For this review, take the finished solid that the model builds, in its own axes (mm). Face numbers are marked on the shaded views. A direction names the side the tool comes from. Round coordinates to 2 decimals unless told otherwise and drop trailing zeros. Order: outer loops, then holes, each group sorted by start corner. A loop starts at its lowest first (then second) coordinate and runs counter-clockwise, first axis right, second up. Notation, with made-up numbers: M 58.5,11 L 98.5,11 A30 ccw 98.5,48 Z; hole C 43,86 d9. An arc over 180 degrees is marked long. Answer in a Markdown table with one row per item. Add a question column.
```python
from build123d import *

# Parameters (mm, degrees)
SKETCH_1_R          = 18
EXTRUDE_1_DEPTH     = 1
SKETCH_2_R          = 8
EXTRUDE_2_DEPTH     = 17
SKETCH_3_R          = 2
EXTRUDE_3_DEPTH     = 3
SKETCH_4_R          = 5
CUT_EXTRUDE_1_DEPTH = 8
SKETCH_5_W          = 4.070351758
SKETCH_5_H          = 5.859394111
CUT_EXTRUDE_2_DEPTH = 0.5


with BuildPart() as part:
    # Эскиз1 → Бобышка-Вытянуть1 (new body)
    with BuildSketch(Plane(origin=(0, 0, 0), x_dir=(1, 0, 0), z_dir=(0, 1, 0))):
        with Locations(Location((0, 0, 0), (0, 0, 270))):
            Circle(SKETCH_1_R)
    extrude(amount=EXTRUDE_1_DEPTH)

    # Эскиз2 → Бобышка-Вытянуть2 (add)
    with BuildSketch(Plane(origin=(0, 1, 0), x_dir=(1, 0, 0), z_dir=(0, 1, 0))):
        with Locations(Location((0, 0, 0), (0, 0, 270))):
            Circle(SKETCH_2_R)
    extrude(amount=EXTRUDE_2_DEPTH)

    # Эскиз3 → Бобышка-Вытянуть3 (add)
    with BuildSketch(Plane(origin=(0, 18, 0), x_dir=(1, 0, 0), z_dir=(0, 1, 0))):
        with Locations(Location((0, 0, 0), (0, 0, 270))):
            Circle(SKETCH_3_R)
    extrude(amount=EXTRUDE_3_DEPTH)

    # Эскиз4 → Вырез-Вытянуть1 (cut)
    with BuildSketch(Plane.XZ):
        with Locations(Location((0, 0, 0), (0, 0, 270))):
            Circle(SKETCH_4_R)
    extrude(amount=-CUT_EXTRUDE_1_DEPTH, mode=Mode.SUBTRACT)

    # Эскиз5 → Вырез-Вытянуть2 (cut)
    with BuildSketch(Plane.XZ):
        with BuildLine():
            Line((-4.012728592, 2.982953109), (-17.751112381, 2.982953109))
            ThreePointArc((-17.751112381, 2.982953109), (-17.937670178, 1.496659138), (-18, 0))
            ThreePointArc((-18, 0), (-17.942077496, -1.442863516), (-17.768682764, -2.876441002))
            Line((-17.768682764, -2.876441002), (-4.089753924, -2.876441002))
            ThreePointArc((-4.089753924, -2.876441002), (-4.999568038, 0.065722391), (-4.012728592, 2.982953109))
        make_face()
        with BuildLine():
            ThreePointArc((18, 0), (17.937670178, 1.496659138), (17.751112381, 2.982953109))
            Line((17.751112381, 2.982953109), (4.012728592, 2.982953109))
            ThreePointArc((4.012728592, 2.982953109), (4.746769584, 1.571043768), (5, 0))
            ThreePointArc((5, 0), (4.767010049, -1.508514232), (4.089753924, -2.876441002))
            Line((4.089753924, -2.876441002), (17.768682764, -2.876441002))
            ThreePointArc((17.768682764, -2.876441002), (17.942077496, -1.442863516), (18, 0))
        make_face()
        with BuildLine():
            Line((-2.035175879, -2.876441002), (-2.035175879, 2.982953109))
            Line((-2.035175879, 2.982953109), (-4.012728592, 2.982953109))
            ThreePointArc((-4.012728592, 2.982953109), (-4.999568038, 0.065722391), (-4.089753924, -2.876441002))
            Line((-4.089753924, -2.876441002), (-2.035175879, -2.876441002))
        make_face()
        with BuildLine():
            Line((4.012728592, 2.982953109), (2.035175879, 2.982953109))
            Line((2.035175879, 2.982953109), (2.035175879, -2.876441002))
            Line((2.035175879, -2.876441002), (4.089753924, -2.876441002))
            ThreePointArc((4.089753924, -2.876441002), (4.767010049, -1.508514232), (5, 0))
            ThreePointArc((5, 0), (4.746769584, 1.571043768), (4.012728592, 2.982953109))
        make_face()
        with BuildLine():
            ThreePointArc((4.012728592, 2.982953109), (3.125961884, 3.902353431), (2.035175879, 4.567062419))
            Line((2.035175879, 4.567062419), (2.035175879, 2.982953109))
            Line((2.035175879, 2.982953109), (4.012728592, 2.982953109))
        make_face()
        with BuildLine():
            ThreePointArc((2.035175879, 4.567062419), (0, 5), (-2.035175879, 4.567062419))
            Line((-2.035175879, 4.567062419), (-2.035175879, 2.982953109))
            Line((-2.035175879, 2.982953109), (2.035175879, 2.982953109))
            Line((2.035175879, 2.982953109), (2.035175879, 4.567062419))
        make_face()
        with BuildLine():
            ThreePointArc((2.035175879, 17.884576012), (1.019223179, 17.971120836), (0, 18))
            ThreePointArc((0, 18), (-1.019223179, 17.971120836), (-2.035175879, 17.884576012))
            Line((-2.035175879, 17.884576012), (-2.035175879, 4.567062419))
            ThreePointArc((-2.035175879, 4.567062419), (0, 5), (2.035175879, 4.567062419))
            Line((2.035175879, 4.567062419), (2.035175879, 17.884576012))
        make_face()
        with BuildLine():
            ThreePointArc((2.035175879, -4.567062419), (0, -5), (-2.035175879, -4.567062419))
            Line((-2.035175879, -4.567062419), (-2.035175879, -17.884576012))
            ThreePointArc((-2.035175879, -17.884576012), (-1.019223179, -17.971120836), (0, -18))
            ThreePointArc((0, -18), (1.019223179, -17.971120836), (2.035175879, -17.884576012))
            Line((2.035175879, -17.884576012), (2.035175879, -4.567062419))
        make_face()
        with Locations((0, 0.053256054)):
            Rectangle(SKETCH_5_W, SKETCH_5_H)
        with BuildLine():
            Line((4.089753924, -2.876441002), (2.035175879, -2.876441002))
            Line((2.035175879, -2.876441002), (2.035175879, -4.567062419))
            ThreePointArc((2.035175879, -4.567062419), (3.176986224, -3.86092716), (4.089753924, -2.876441002))
        make_face()
        with BuildLine():
            Line((2.035175879, -2.876441002), (-2.035175879, -2.876441002))
            Line((-2.035175879, -2.876441002), (-2.035175879, -4.567062419))
            ThreePointArc((-2.035175879, -4.567062419), (0, -5), (2.035175879, -4.567062419))
            Line((2.035175879, -4.567062419), (2.035175879, -2.876441002))
        make_face()
        with BuildLine():
            Line((-2.035175879, -4.567062419), (-2.035175879, -2.876441002))
            Line((-2.035175879, -2.876441002), (-4.089753924, -2.876441002))
            ThreePointArc((-4.089753924, -2.876441002), (-3.176986224, -3.86092716), (-2.035175879, -4.567062419))
        make_face()
        with BuildLine():
            Line((-2.035175879, 2.982953109), (-2.035175879, 4.567062419))
            ThreePointArc((-2.035175879, 4.567062419), (-3.125961884, 3.902353431), (-4.012728592, 2.982953109))
            Line((-4.012728592, 2.982953109), (-2.035175879, 2.982953109))
        make_face()
    extrude(amount=-CUT_EXTRUDE_2_DEPTH, mode=Mode.SUBTRACT)


solid = part.part
```
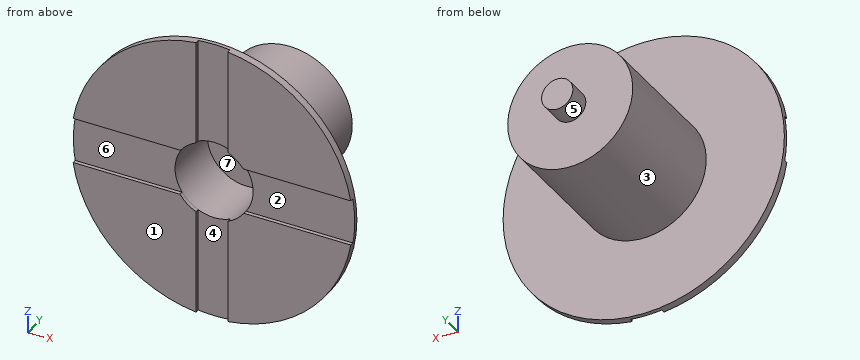
1. The part is to be moulded in two halves that separate along Z. For the marked faces 1, 2 and 3, say which applies: pulls with the +Z half, pulls with the -Z half, needs draft (parallel to the pull), parting line crosses it, or undercut.
2. Consider section A-A on x = 0. Write out the cut boundary in (y, z), plus the area to 3 significant figures.
3. To check wall thickness, follow probe 1 along X at (y, z) = (4.5, 0); probe 2 along Y at (x, z) = (-7.5, -6); probe 3 along Y at (x, z) = (-2.5, -2). State the ranges of each line that lie inside material, in increasing order. Write a range as [from, to].
4. Consider section D-D on y = 15.5. Write out the cut boundary in (x, z), plus the area to 3 significant figures.
5. Consider section C-C on z = 0. Write out the cut boundary in (x, y).
6. For the marked faces 4, 5, 6 and 7, list the 3-axis set-ups (+Z, -Z, +X, -X, +Y, -Y) from which the entire face can be reached by the end or side of a thin tool; tool diameter is ignored.
7. Clearance check with flat-ended pins moving along their axes: pin 1 Ø3 at (x, z) = (1.5, -2) entering from -Y; pin 2 Ø1.5 at (x, z) = (1.5, -4) entering from +Y; pin 3 Ø12 at (x, y) = (4.5, 16.5) entering from -Z. State where each tip first meets the part, or that it passes through.
8. Consider section B-B on y = 4.5. Write out the cut boundary in (x, z), plus the area to 3 significant figures.
Solved:
| question | item | result |
|---|---|---|
| 1 | face 1 | needs draft |
| 1 | face 2 | undercut |
| 1 | face 3 | parting line crosses it |
| 2 | outline | M 0.5,-18 L 1,-18 L 1,-8 L 18,-8 L 18,-2 L 21,-2 L 21,2 L 18,2 L 18,8 L 1,8 L 1,18 L 0.5,18 L 0.5,5 L 8,5 L 8,-5 L 0.5,-5 Z |
| 2 | area | 227 mm^2 |
| 3 | probe 1 | x = [-8, -5], [5, 8] |
| 3 | probe 2 | y = [0, 1] |
| 3 | probe 3 | y = [8, 18] |
| 4 | outline | C 0,0 d16 |
| 4 | area | 201 mm^2 |
| 5 | outline | M -18,0.5 L -5,0.5 L -5,8 L 5,8 L 5,0.5 L 18,0.5 L 18,1 L 8,1 L 8,18 L 2,18 L 2,21 L -2,21 L -2,18 L -8,18 L -8,1 L -18,1 Z |
| 6 | face 4 | +Z, -Z, -Y |
| 6 | face 5 | +Y |
| 6 | face 6 | +X, -X, -Y |
| 6 | face 7 | -Y |
| 7 | pin 1 | stops at y = 8 |
| 7 | pin 2 | stops at y = 18 |
| 7 | pin 3 | stops at z = -8 |
| 8 | outline | C 0,0 d16; hole C 0,0 d10 |
| 8 | area | 123 mm^2 |
